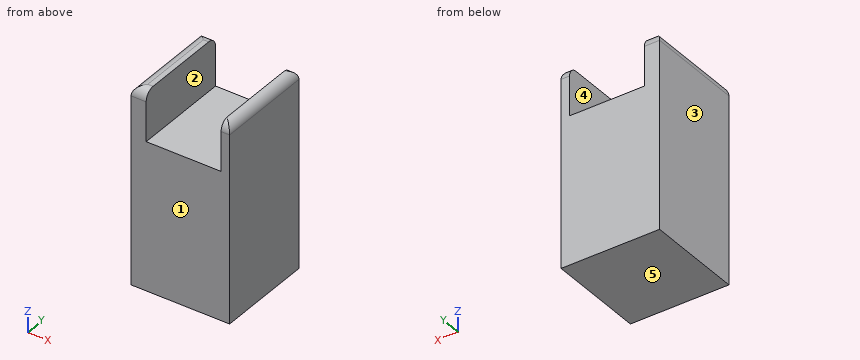
from build123d import *

# Parameters (mm, degrees)
F0_W     = 50
F0_H     = 100
F1_DEPTH = 50
F2_R     = 5
F4_W     = 38
F4_H     = 53.0364588497
F5_DEPTH = 25


with BuildPart() as f1:
    # F0 (on Front) → F1 (new body)
    with BuildSketch(Plane.XZ):
        with Locations((-43.9743227283, -14.4022647291)):
            Rectangle(F0_W, F0_H)
    extrude(amount=F1_DEPTH)

    # F2
    f2_edges = [f1.edges().sort_by_distance(p)[0] for p in [
        (-18.974323, -25, 35.597735),
        (-68.974323, -25, 35.597735),
        (-43.974323, 0, 35.597735),
        (-43.974323, -50, 35.597735),
    ]]
    fillet(f2_edges, radius=F2_R)

    # F4 (on face) → F5 (cut)
    with BuildSketch(Plane.XY.offset(35.5977352709)):
        with Locations((-42.2953676743, -26.5182294249)):
            Rectangle(F4_W, F4_H)
    extrude(amount=-F5_DEPTH, mode=Mode.SUBTRACT)


solid = f1.part
The listing builds one solid part. Answer for the finished solid, in the listing's coordinates (mm). Face numbers are marked on the shaded views. A direction names the side the tool comes from. Coordinates: 2 decimals unless noted, no trailing zeros. Write each loop counter-clockwise with the first axis right and the second up, starting at its lowest first coordinate (ties: lowest second). Pieces come first, ordered by that corner, then holes. Notation, with made-up numbers: (17.25, 89) - (65.25, 89) arc R35 cw to (65.25, 126) - close; hole circle Ø7 at (59, 13.25). An arc over 180 degrees is marked (long way). Answer as CSV lines item,"result".
1. A tool of negligible diameter and unlimited length cuts with its end or side. For the marked faces 1 and 2, from which of +Z, -Z, +X, -X, +Y, -Y can it reach the whole face along a straight path? Write none if from no direction.
Computed values:
face 1,"+Z, -Z, +X, -X, -Y"
face 2,"+Z, +Y, -Y"
2. Find section B-B (x = -27.5). Give the vertices of the cut face in (y, z), plus the area to 3 significant figures.
Computed values:
outline,"(-50, -64.4) - (0, -64.4) - (0, 10.6) - (-50, 10.6) - close"
area,"3,750 mm²"
3. Straight lines are drawn through the part: line 1 (X direction, y = -39, z = 11.5); line 2 (Z direction, x = -37, y = -41); line 3 (Z direction, x = -23, y = -44). For each, find the intervals that lie inside material, in ascending order. Write a range as [from, to].
Computed values:
line 1,"x = [-68.97, -61.3], [-23.3, -18.97]"
line 2,"z = [-64.4, 10.6]"
line 3,"z = [-64.4, 35.5]"
4. Determine the mould class of the marked faces 3, 4 and 5 for opening direction X: +X half, -X half, draft (parallel to the pull), parting line (faces both ways), or undercut.
Computed values:
face 3,"-X half"
face 4,"undercut"
face 5,"draft"
5. Find section A-A (y = -26). Give the vertices of the cut face in (x, z).
Computed values:
outline,"(-68.97, -64.4) - (-18.97, -64.4) - (-18.97, 30.6) arc R5 ccw to (-23.3, 35.55) - (-23.3, 10.6) - (-61.3, 10.6) - (-61.3, 35.6) - (-63.97, 35.6) arc R5 ccw to (-68.97, 30.6) - close"
